Verification items for the finished model (mm, model axes). Round coordinates to 2 decimals unless told otherwise and drop trailing zeros. Loops run counter-clockwise (first coordinate to the right, second up) from the corner with the lowest first, then second, coordinate; pieces in that order, holes last.
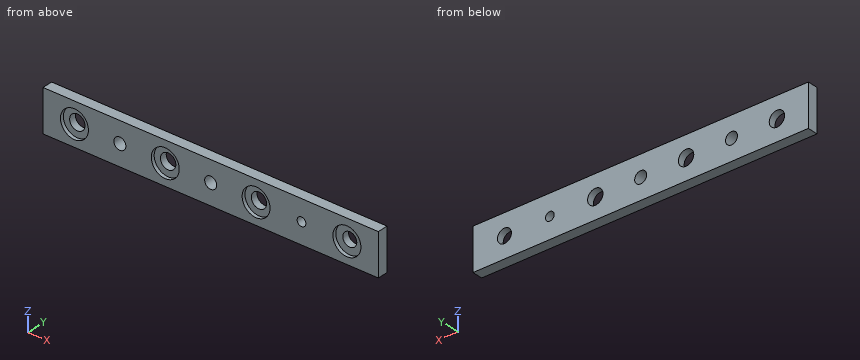
from build123d import *

# Parameters (mm, degrees)
F0_W     = 304.8
F0_H     = 38.1
F0_R     = 6.985
F0_R_2   = 6.35
F1_DEPTH = 9.525
F2_R     = 5.461
F2_R_2   = 3.96875
F3_DEPTH = 9.526
F2_R_3   = 12.7
F2_R_4   = 6.985
F2_R_5   = 6.35
F4_DEPTH = 3.175


with BuildPart() as f1:
    # F0 (on Front) → F1 (new body)
    with BuildSketch(Plane.XZ):
        with Locations((152.4, 19.05)):
            Rectangle(F0_W, F0_H)
        with Locations((28.575, 19.05)):
            Circle(F0_R, mode=Mode.SUBTRACT)
        with Locations((111.125, 19.05)):
            Circle(F0_R, mode=Mode.SUBTRACT)
        with Locations((193.675, 19.05)):
            Circle(F0_R, mode=Mode.SUBTRACT)
        with Locations((276.225, 19.05)):
            Circle(F0_R_2, mode=Mode.SUBTRACT)
    extrude(amount=F1_DEPTH)

    # F2 (on face) → F3 (cut, through all)
    with BuildSketch(Plane.XZ.offset(9.525)):
        with Locations((69.85, 19.05)):
            Circle(F2_R)
        with Locations((152.4, 19.05)):
            Circle(F2_R)
        with Locations((234.95, 19.05)):
            Circle(F2_R_2)
    extrude(amount=-F3_DEPTH, mode=Mode.SUBTRACT)

    # F2 (on face) → F4 (cut)
    with BuildSketch(Plane.XZ.offset(9.525)):
        with Locations((28.575, 19.05)):
            Circle(F2_R_3)
        with Locations((28.575, 19.05)):
            Circle(F2_R_4, mode=Mode.SUBTRACT)
        with Locations((111.125, 19.05)):
            Circle(F2_R_3)
        with Locations((111.125, 19.05)):
            Circle(F2_R_4, mode=Mode.SUBTRACT)
        with Locations((193.675, 19.05)):
            Circle(F2_R_3)
        with Locations((193.675, 19.05)):
            Circle(F2_R_4, mode=Mode.SUBTRACT)
        with Locations((276.225, 19.05)):
            Circle(F2_R_3)
        with Locations((276.225, 19.05)):
            Circle(F2_R_5, mode=Mode.SUBTRACT)
    extrude(amount=-F4_DEPTH, mode=Mode.SUBTRACT)


solid = f1.part
1. Section check A-A (x = 234.95). Enter the section's corners in (y, z) (3 decimals).
2. Section check B-B (y = -2.75). Give the number of separate pieces and of enclosed holes in the cut face, then the cut area to 3 significant figures.
3. Section check D-D (z = 9.5). Enter the section's corners in (x, y) (3 decimals).
4. Section check C-C (x = 152.4). Enter the section's corners in (y, z) (3 decimals).
5. Gauge pin test, flat ends, axial feed: P1, Ø10, axis at x = 69.85, z = 19.05, coming from the +Y side; P2, Ø16, axis at x = 28.575, z = 19.05, coming from the -Y side. Record the tip position at first contact, or that the pin passes through.
6. Scan lines: L1, parallel to Z at x = 69.85, y = -2.5; L2, parallel to X at y = -6.5, z = 10.5; L3, parallel to Z at x = 106.5, y = -6.25. Record each from-to range of solid material in increasing order.
Taken from the geometry:
1. outline: (-9.525, 0) - (0, 0) - (0, 15.081) - (-9.525, 15.081) - close; (-9.525, 23.019) - (0, 23.019) - (0, 38.1) - (-9.525, 38.1) - close
2. separate pieces: 1
2. enclosed holes: 7
2. area: 10,800 mm2
3. outline: (0, -9.525) - (20.203, -9.525) - (20.203, -6.35) - (36.947, -6.35) - (36.947, -9.525) - (102.753, -9.525) - (102.753, -6.35) - (119.497, -6.35) - (119.497, -9.525) - (185.303, -9.525) - (185.303, -6.35) - (202.047, -6.35) - (202.047, -9.525) - (267.853, -9.525) - (267.853, -6.35) - (284.597, -6.35) - (284.597, -9.525) - (304.8, -9.525) - (304.8, 0) - (0, 0) - close
4. outline: (-9.525, 0) - (0, 0) - (0, 13.589) - (-9.525, 13.589) - close; (-9.525, 24.511) - (0, 24.511) - (0, 38.1) - (-9.525, 38.1) - close
5. P1: passes through
5. P2: stops at y = -6.35
6. L1: z = 0 to 13.59, 24.51 to 38.1
6. L2: x = 0 to 19.18, 37.97 to 101.73, 120.52 to 184.28, 203.07 to 266.83, 285.62 to 304.8
6. L3: z = 0 to 13.82, 24.28 to 38.1
